The model under review builds one solid part; all positions refer to its coordinate system, in mm. Coordinates: 2 decimals unless noted, no trailing zeros. Write each loop counter-clockwise with the first axis right and the second up, starting at its lowest first coordinate (ties: lowest second). Pieces come first, ordered by that corner, then holes. Notation, with made-up numbers: M 60,83 L 80,83 A22 ccw 80,117 Z; hole C -1,15.5 d5. An arc over 180 degrees is marked long. Answer as a JSON object with one key per item and string values.
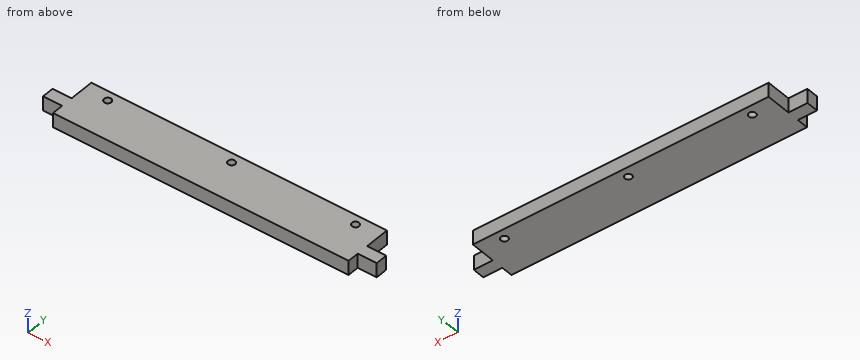
```python
from build123d import *

# Parameters (mm, degrees)
SKETCH_1_W          = 124
SKETCH_1_H          = 20.28
EXTRUDE_1_DEPTH     = 6
SKETCH_2_W          = 8
SKETCH_2_H          = 5
EXTRUDE_2_DEPTH     = 6
SKETCH_3_R          = 1.5
CUT_EXTRUDE_1_DEPTH = 134.683500852


with BuildPart() as part:
    # 草图1 → 凸台-拉伸1 (new body)
    with BuildSketch(Plane.XY):
        with Locations((62, 10.14)):
            Rectangle(SKETCH_1_W, SKETCH_1_H)
    extrude(amount=EXTRUDE_1_DEPTH)

    # 草图2 → 凸台-拉伸2 (add)
    with BuildSketch(Plane.XY.offset(6)):
        with Locations((-4, 7.28)):
            Rectangle(SKETCH_2_W, SKETCH_2_H)
        with Locations((128, 7.28)):
            Rectangle(SKETCH_2_W, SKETCH_2_H)
    extrude(amount=-EXTRUDE_2_DEPTH)

    # 草图3 → 切除-拉伸1 (cut, through all)
    with BuildSketch(Plane(origin=(0, 0, 0), x_dir=(-1, 0, 0), z_dir=(0, 0, -1))):
        with Locations((-62, 16.28)):
            Circle(SKETCH_3_R)
        with Locations((-114, 16.28)):
            Circle(SKETCH_3_R)
        with Locations((-10, 16.28)):
            Circle(SKETCH_3_R)
    extrude(amount=-CUT_EXTRUDE_1_DEPTH, mode=Mode.SUBTRACT)


solid = part.part
```
(1) Wall thickness on line 1 along Y through (x, z) = (10, 3.7); line 2 along X through (y, z) = (17.5, 2.9); line 3 along X through (y, z) = (12.5, 2.95): over which ranges is each line inside the solid? List them lowest first. Write a range as from..to.
Results list:
{"line 1": "0..14.78, 17.78..20.28", "line 2": "0..9.13, 10.87..61.13, 62.87..113.13, 114.87..124", "line 3": "0..124"}
(2) Add section A-A on y = 16.28. Give the boundary of the cut face in (x, z), and give its area (3 significant figures).
Results list:
{"outline": "M 0,0 L 8.5,0 L 8.5,6 L 0,6 Z; M 11.5,0 L 60.5,0 L 60.5,6 L 11.5,6 Z; M 63.5,0 L 112.5,0 L 112.5,6 L 63.5,6 Z; M 115.5,0 L 124,0 L 124,6 L 115.5,6 Z", "area": "690 mm²"}
(3) Add section B-B on z = 3.6. Give the boundary of the cut face in (x, y), and give its area (3 significant figures).
Results list:
{"outline": "M -8,4.78 L 0,4.78 L 0,0 L 124,0 L 124,4.78 L 132,4.78 L 132,9.78 L 124,9.78 L 124,20.28 L 0,20.28 L 0,9.78 L -8,9.78 Z; hole C 10,16.28 d3; hole C 62,16.28 d3; hole C 114,16.28 d3", "area": "2,570 mm²"}
(4) Add section C-C on x = 62. Give the boundary of the cut face in (y, z), and give its area (3 significant figures).
Results list:
{"outline": "M 0,0 L 14.78,0 L 14.78,6 L 0,6 Z; M 17.78,0 L 20.28,0 L 20.28,6 L 17.78,6 Z", "area": "104 mm²"}
(5) For pin 1 Ø1.8 at (x, z) = (-2.5, 3.5) entering from +Y; pin 2 Ø1 at (y, z) = (14.5, 4.5) entering from +X; pin 3 Ø3 at (x, z) = (126.5, 2) entering from -Y, all flat-tipped, find the tip position at first contact; note any pin that passes through.
Results list:
{"pin 1": "y = 9.78", "pin 2": "x = 124", "pin 3": "y = 4.78"}
